Print and shaded views of the part. All mm, measured from the part's lowest x, y and z. A direction names the side the tool comes from. Round coordinates to 2 decimals unless told otherwise and drop trailing zeros. Loops run counter-clockwise (first coordinate to the right, second up) from the corner with the lowest first, then second, coordinate; pieces in that order, holes last. Notation, with made-up numbers: (51, 60.25) - (66, 60.25) arc R14 ccw to (66, 65.25) - close; hole circle Ø8 at (49.25, 4.5). An arc over 180 degrees is marked (long way). Use one line per item in the form item = value.
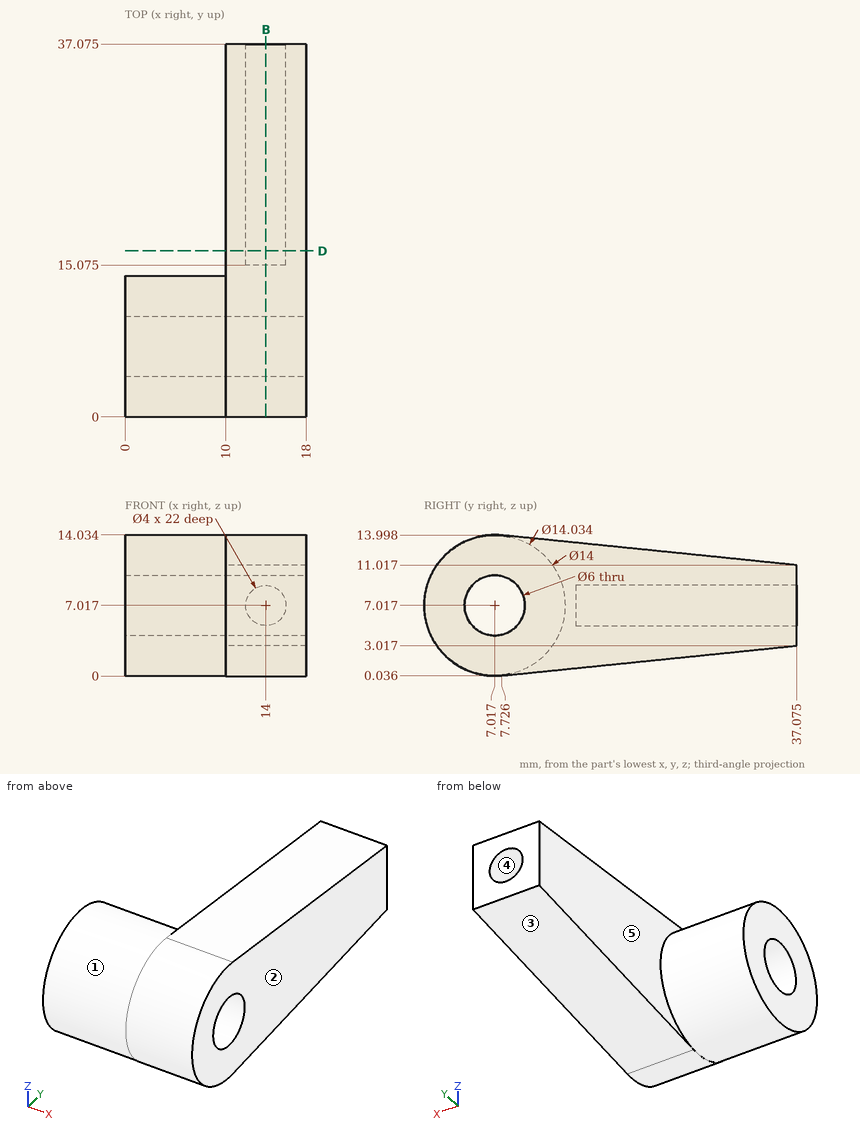
1) Tool access for the marked faces 1 and 2: list every direction of +Z, -Z, +X, -X, +Y, -Y with a clear straight run to the whole face (end or side of a thin tool).
Report:
face_1 = -X
face_2 = +Z, -Z, +X, +Y, -Y
2) Slice it at B-B (x = 14). Write the cut outline in (y, z) (1 decimal).
Report:
outline = (7.7, 0) - (37.1, 3) - (37.1, 5) - (15.1, 5) - (15.1, 9) - (37.1, 9) - (37.1, 11) - (7.7, 14) arc R7 ccw (long way) to start; hole circle Ø6 at (7, 7)
3) Slice it at D-D (y = 16.5). Write the cut outline in (x, z).
Report:
outline = (10, 0.93) - (18, 0.93) - (18, 13.11) - (10, 13.11) - close; hole circle Ø4 at (14, 7.02)
4) Drill centre lines: probe 1 along X at (y, z) = (15, 4.25); probe 2 along Y at (x, z) = (8.25, 6) (1 decimal); probe 3 along X at (y, z) = (23.5, 8.25) (1 decimal). Where is each one in solid material? Low to high.
Report:
probe_1 = 10 to 18
probe_2 = 0.1 to 4.2, 9.8 to 13.9
probe_3 = 10 to 12.4, 15.6 to 18
5) Flat gauge pins, fed straight in: pin 1 (4 mm diameter, centred on x = 2.5, z = 3.5, fed in from -Y); pin 2 (5 mm diameter, centred on x = 15, y = 31.5, fed in from -Z); pin 3 (2 mm diameter, centred on x = 2, y = 9, fed in from -Z); pin 4 (4.5 mm diameter, centred on x = 14, z = 7, fed in from +Y) (3 decimals). Where does each tip first touch, or does it go through?
Report:
pin_1 = 0.18
pin_2 = 2.2
pin_3 = 0.09
pin_4 = 37.075
6) Two-plate mould, pull along X, no slides. Class the marked faces 3, 4 and 5: +X half, -X half, draft (parallel to the pull), parting line (faces both ways), or undercut.
Report:
face_3 = draft
face_4 = undercut
face_5 = -X half
